The listing builds one solid part. Answer for the finished solid, in the listing's coordinates (mm). A direction names the side the tool comes from. Give positions to 0.01 mm unless a question says otherwise; leave off trailing zeros. Order: outer loops, then holes, each group sorted by start corner. A loop starts at its lowest first (then second) coordinate and runs counter-clockwise, first axis right, second up. Notation, with made-up numbers: M -3.75,85.25 L 19.25,85.25 A13 cw 19.25,109.25 Z; hole C 2.25,66 d9. An arc over 180 degrees is marked long. Answer as a JSON object with one key per item and string values. Group by question number.
```python
from build123d import *

# Parameters (mm, degrees)
SKETCH_1_W          = 32
SKETCH_1_H          = 18.6
EXTRUDE_1_DEPTH     = 2.2
FILLET_1_R          = 2
SKETCH_2_W          = 3.14
SKETCH_2_H          = 10.76
SKETCH_2_W_2        = 16.8
SKETCH_2_H_2        = 2.6
CUT_EXTRUDE_1_DEPTH = 3.2
EXTRUDE_2_DEPTH     = 0.7
CHAMFER_1_SIZE      = 0.3
CHAMFER_2_SIZE      = 1


with BuildPart() as part:
    # 草图1 → 凸台-拉伸1 (new body)
    with BuildSketch(Plane(origin=(0, 0, 0), x_dir=(1, 0, 0), z_dir=(0, 1, 0))):
        with Locations((47.27991, 9.3)):
            Rectangle(SKETCH_1_W, SKETCH_1_H)
    extrude(amount=EXTRUDE_1_DEPTH)

    # 圆角1
    fillet_1_edges = [part.edges().sort_by_distance(p)[0] for p in [
        (31.27991, 1.1, -18.6),
        (63.27991, 1.1, -18.6),
        (63.27991, 1.1, 0),
        (31.27991, 1.1, 0),
    ]]
    fillet(fillet_1_edges, radius=FILLET_1_R)

    # 草图2 → 切除-拉伸1 (cut, through all)
    with BuildSketch(Plane(origin=(0, 2.2, 0), x_dir=(1, 0, 0), z_dir=(0, 1, 0))):
        with Locations((34.54991, 11.32)):
            Rectangle(SKETCH_2_W, SKETCH_2_H)
        with Locations((51.17991, 1)):
            Rectangle(SKETCH_2_W_2, SKETCH_2_H_2)
        with Locations((51.17991, 17.6)):
            Rectangle(SKETCH_2_W_2, SKETCH_2_H_2)
    extrude(amount=-CUT_EXTRUDE_1_DEPTH, mode=Mode.SUBTRACT)

    # 草图3 → 凸台-拉伸2 (add)
    with BuildSketch(Plane.XZ):
        with BuildLine():
            Line((36.11991, -5.94), (36.11991, -2.3))
            Line((36.11991, -2.3), (42.77991, -2.3))
            Line((42.77991, -2.3), (42.77991, 0))
            Line((42.77991, 0), (33.27991, 0))
            ThreePointArc((33.27991, 0), (31.865696, -0.585786), (31.27991, -2))
            Line((31.27991, -2), (31.27991, -16.6))
            ThreePointArc((31.27991, -16.6), (31.865696, -18.014214), (33.27991, -18.6))
            Line((33.27991, -18.6), (42.77991, -18.6))
            Line((42.77991, -18.6), (42.77991, -16.3))
            Line((42.77991, -16.3), (36.11991, -16.3))
            Line((36.11991, -16.3), (36.11991, -16.7))
            Line((36.11991, -16.7), (32.97991, -16.7))
            Line((32.97991, -16.7), (32.97991, -5.94))
            Line((32.97991, -5.94), (36.11991, -5.94))
        make_face()
        with BuildLine():
            Line((59.57991, -16.3), (59.57991, -18.6))
            Line((59.57991, -18.6), (61.27991, -18.6))
            ThreePointArc((61.27991, -18.6), (62.694123, -18.014214), (63.27991, -16.6))
            Line((63.27991, -16.6), (63.27991, -2))
            ThreePointArc((63.27991, -2), (62.694123, -0.585786), (61.27991, 0))
            Line((61.27991, 0), (59.57991, 0))
            Line((59.57991, 0), (59.57991, -2.3))
            Line((59.57991, -2.3), (59.57991, -16.3))
        make_face()
    extrude(amount=EXTRUDE_2_DEPTH)

    # 倒角1
    chamfer_1_edges = [part.edges().sort_by_distance(p)[0] for p in [
        (36.11991, -0.7, -4.12),
        (34.54991, -0.7, -5.94),
        (39.44991, -0.7, -16.3),
        (42.77991, -0.7, -17.45),
        (38.02991, -0.7, -18.6),
        (31.865696, -0.7, -18.014214),
        (31.27991, -0.7, -9.3),
        (31.865696, -0.7, -0.585786),
        (38.02991, -0.7, 0),
        (42.77991, -0.7, -1.15),
        (39.44991, -0.7, -2.3),
        (60.42991, -0.7, 0),
        (62.694123, -0.7, -0.585786),
        (63.27991, -0.7, -9.3),
        (62.694123, -0.7, -18.014214),
        (60.42991, -0.7, -18.6),
        (59.57991, -0.7, -9.3),
        (38.02991, 2.2, 0),
        (31.865696, 2.2, -0.585786),
        (31.27991, 2.2, -9.3),
        (31.865696, 2.2, -18.014214),
        (38.02991, 2.2, -18.6),
        (42.77991, 2.2, -17.45),
        (51.17991, 2.2, -16.3),
        (59.57991, 2.2, -17.45),
        (60.42991, 2.2, -18.6),
        (62.694123, 2.2, -18.014214),
        (63.27991, 2.2, -9.3),
        (62.694123, 2.2, -0.585786),
        (60.42991, 2.2, 0),
        (59.57991, 2.2, -1.15),
        (51.17991, 2.2, -2.3),
        (42.77991, 2.2, -1.15),
        (34.54991, 2.2, -16.7),
        (32.97991, 2.2, -11.32),
        (34.54991, 2.2, -5.94),
        (36.11991, 2.2, -11.32),
        (42.77991, 0.75, -18.6),
        (42.77991, 1.1, -16.3),
        (59.57991, 1.1, -16.3),
        (59.57991, 0.75, -18.6),
        (59.57991, 0.75, 0),
        (59.57991, 1.1, -2.3),
        (42.77991, 1.1, -2.3),
        (42.77991, 0.75, 0),
    ]]
    chamfer(chamfer_1_edges, length=CHAMFER_1_SIZE)

    # 倒角2
    chamfer_2_edges = [part.edges().sort_by_distance(p)[0] for p in [
        (32.97991, -0.7, -11.32),
    ]]
    chamfer(chamfer_2_edges, length=CHAMFER_2_SIZE)


solid = part.part
```
Item 1: A tool of negligible diameter and unlimited length cuts with its end or side. For faces 5 (the flat face through (38, 1, 0)), 6 (the flat face through (36.12, 1, -11)), 7 (the flat face through (51, 1, -2.3)), 8 (the flat face through (51, 1, -16.3)), 9 (the conical face through (31.98, 2.08, -0.73)), from which of +Z, -Z, +X, -X, +Y, -Y can it reach the whole face along a straight path? Write none if from no direction.
Item 2: Flat-ended cylindrical pins translate along their axes: P1, Ø6, axis at x = 51, z = -14.5, coming from the -Y side; P2, Ø1.5, axis at x = 52, y = 1.5, coming from the +Z side. Find the tip coordinate at first contact, or state that the pin passes through.
Item 3: Section D-D (z = -4.5) is taken. Determine the outline of the cut face in (x, y).
Item 4: Section A-A (x = 41.5) is taken. Determine the outline of the cut face in (y, z).
Item 5: Consider probe 1 along X at (y, z) = (0.65, -10.75); probe 2 along Y at (x, z) = (41, -8.5); probe 3 along Z at (x, y) = (49, 0.05). Determine where each line is inside the solid, lowest interval first. Write a range as from..to.
Item 6: Section C-C (y = 0.95) is taken. Determine the outline of the cut face in (x, z).
Item 7: Section B-B (z = -7.25) is taken. Determine the outline of the cut face in (x, y), and give its area (3 significant figures).
Item 8: Determine the mould class of faces 1 (the flat face through (48, 0, -9)), 2 (the conical face through (32.01, -0.58, -0.7)), 3 (the conical face through (62.55, 2.08, -17.9)), 4 (the flat face through (32.98, 1, -11)) for opening direction X: released by +X, released by -X, zero draft, split by the parting line, or undercut.
Values found:
{
 "1": {"face 5": "+Z, +X, -X, +Y, -Y", "face 6": "+Y, -Y", "face 7": "+Z, +Y, -Y", "face 8": "-Z, +Y, -Y", "face 9": "+Z, -X, +Y"},
 "2": {"P1": "stops at y = 0", "P2": "stops at z = -2.3"},
 "3": {"outline": "M 31.28,-0.4 L 31.58,-0.7 L 35.82,-0.7 L 36.12,-0.4 L 36.12,0 L 59.58,0 L 59.58,-0.4 L 59.88,-0.7 L 62.98,-0.7 L 63.28,-0.4 L 63.28,1.9 L 62.98,2.2 L 31.58,2.2 L 31.28,1.9 Z"},
 "4": {"outline": "M -0.7,-18.3 L -0.4,-18.6 L 1.9,-18.6 L 2.2,-18.3 L 2.2,-0.3 L 1.9,0 L -0.4,0 L -0.7,-0.3 L -0.7,-2 L -0.4,-2.3 L 0,-2.3 L 0,-16.3 L -0.4,-16.3 L -0.7,-16.6 Z"},
 "5": {"probe 1": "x = 31.28..32.98, 36.12..63.28", "probe 2": "y = 0..2.2", "probe 3": "z = -16.3..-2.3"},
 "6": {"outline": "M 31.28,-16.6 A2 ccw 33.28,-18.6 L 42.48,-18.6 L 42.78,-18.3 L 42.78,-16.6 L 43.08,-16.3 L 59.28,-16.3 L 59.58,-16.6 L 59.58,-18.3 L 59.88,-18.6 L 61.28,-18.6 A2 ccw 63.28,-16.6 L 63.28,-2 A2 ccw 61.28,0 L 59.88,0 L 59.58,-0.3 L 59.58,-2 L 59.28,-2.3 L 43.08,-2.3 L 42.78,-2 L 42.78,-0.3 L 42.48,0 L 33.28,0 A2 ccw 31.28,-2 Z; hole M 32.98,-16.7 L 36.12,-16.7 L 36.12,-5.94 L 32.98,-5.94 Z"},
 "7": {"outline": "M 31.28,-0.4 L 31.58,-0.7 L 31.98,-0.7 L 32.98,0.3 L 32.98,1.9 L 32.68,2.2 L 31.58,2.2 L 31.28,1.9 Z; M 36.12,0 L 59.58,0 L 59.58,-0.4 L 59.88,-0.7 L 62.98,-0.7 L 63.28,-0.4 L 63.28,1.9 L 62.98,2.2 L 36.42,2.2 L 36.12,1.9 Z", "area": "66.5 mm^2"},
 "8": {"face 1": "undercut", "face 2": "released by -X", "face 3": "released by +X", "face 4": "undercut"}
}
